For this review, take the finished solid that the model builds, in its own axes (mm). Face numbers are marked on the shaded views. Round coordinates to 2 decimals unless told otherwise and drop trailing zeros. Loops run counter-clockwise (first coordinate to the right, second up) from the corner with the lowest first, then second, coordinate; pieces in that order, holes last. Notation, with made-up numbers: (-14.75, -23) -> (28.25, -23) arc R20 ccw to (28.25, 8) -> close; hole circle Ø2 at (-13.5, -18). An arc over 180 degrees is marked (long way). Write each question's results on one line, items separated by ' | '.
```python
from build123d import *

# Parameters (mm, degrees)
BOSS_EXTRUDE1_DEPTH      = 3.75
BOSS_EXTRUDE1_DEPTH_BACK = 3.75
SKETCH1_R                = 1.5
SKETCH3_R                = 1.5
CUT_EXTRUDE1_DEPTH       = 25.5
SKETCH4_R                = 2.75
CUT_EXTRUDE2_DEPTH       = 25
CUT_EXTRUDE3_DEPTH       = 25
CUT_EXTRUDE4_DEPTH       = 3


with BuildPart() as part:
    # Sketch1 → Boss-Extrude1 (new, two sides: drawn at the far end of the back side and taken through both)
    with BuildSketch(Plane(origin=(0, 0, 0), x_dir=(0, 0, -1), z_dir=(1, 0, 0)).offset(-BOSS_EXTRUDE1_DEPTH_BACK)):
        with BuildLine():
            Line((0, 26), (0, 36))
            ThreePointArc((0, 36), (-36, 0), (0, -36))
            Line((0, -36), (0, -26))
            ThreePointArc((0, -26), (-24.020867845, -9.949769241), (-18.384776311, 18.384776311))
            ThreePointArc((-18.384776311, 18.384776311), (-9.949769241, 24.020867845), (0, 26))
        make_face()
        with Locations((-19.798989873, -19.798989873)):
            Circle(SKETCH1_R, mode=Mode.SUBTRACT)
        with BuildLine():
            ThreePointArc((-18.298989873, 19.798989873), (-18.413170574, 19.224964725), (-18.738329701, 18.738329701))
            ThreePointArc((-18.738329701, 18.738329701), (-21.184809172, 20.373015022), (-18.298989873, 19.798989873))
        make_face(mode=Mode.SUBTRACT)
    extrude(amount=BOSS_EXTRUDE1_DEPTH + BOSS_EXTRUDE1_DEPTH_BACK)

    # Sketch3 → Cut-Extrude1 (cut)
    with BuildSketch(Plane(origin=(0, 0, 0), x_dir=(-1, 0, 0), z_dir=(0, 0, -1))):
        with Locations((0, 31)):
            Circle(SKETCH3_R)
    cut_extrude1 = extrude(amount=-CUT_EXTRUDE1_DEPTH, mode=Mode.SUBTRACT)

    # Mirror1: Cut-Extrude1 across plane
    add(cut_extrude1.mirror(Plane.ZX), mode=Mode.SUBTRACT)

    # Sketch4 → Cut-Extrude2 (cut)
    with BuildSketch(Plane(origin=(0, 0, 30), x_dir=(-1, 0, 0), z_dir=(0, 0, -1))):
        with Locations(Location((0, 31, 0), (0, 0, 180))):
            Circle(SKETCH4_R)
    extrude(amount=CUT_EXTRUDE2_DEPTH, mode=Mode.SUBTRACT)

    # Sketch5 → Cut-Extrude3 (cut)
    with BuildSketch(Plane(origin=(0, 0, 30), x_dir=(-1, 0, 0), z_dir=(0, 0, -1))):
        Polygon((2.75, -32.58771324), (2.75, -29.41228676), (0, -27.824573519), (-2.75, -29.41228676), (-2.75, -32.58771324), (0, -34.175426481), align=None)
    extrude(amount=CUT_EXTRUDE3_DEPTH, mode=Mode.SUBTRACT)

    # Sketch6 → Cut-Extrude4 (cut)
    with BuildSketch(Plane(origin=(3.75, 0, 0), x_dir=(0, 0, -1), z_dir=(1, 0, 0))):
        Polygon((-22.45221952, -18.054367916), (-22.636491632, -21.224443171), (-19.983261985, -22.969065128), (-17.145760226, -21.543611831), (-16.961488115, -18.373536576), (-19.614717761, -16.628914618), align=None)
        Polygon((-18.054367916, 22.45221952), (-21.224443171, 22.636491632), (-22.969065128, 19.983261985), (-21.543611831, 17.145760226), (-18.373536576, 16.961488115), (-16.628914618, 19.614717761), align=None)
        Polygon((18.054367916, -22.45221952), (21.224443171, -22.636491632), (22.969065128, -19.983261985), (21.543611831, -17.145760226), (18.373536576, -16.961488115), (16.628914618, -19.614717761), align=None)
        Polygon((22.45221952, 18.054367916), (22.636491632, 21.224443171), (19.983261985, 22.969065128), (17.145760226, 21.543611831), (16.961488115, 18.373536576), (19.614717761, 16.628914618), align=None)
    extrude(amount=-CUT_EXTRUDE4_DEPTH, mode=Mode.SUBTRACT)


solid = part.part
```
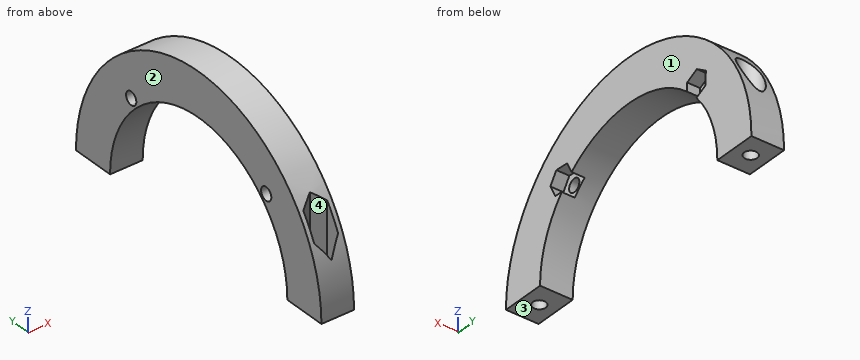
1. Consider section A-A (z = 9). State the section outline as (x, y) points, plus the area to 3 significant figures.
Values found:
outline: (-3.75, -34.86) -> (3.75, -34.86) -> (3.75, -24.39) -> (-3.75, -24.39) -> close; (-3.75, 24.39) -> (3.75, 24.39) -> (3.75, 34.86) -> (-3.75, 34.86) -> close; hole (-2.75, -32.59) -> (0, -34.18) -> (2.75, -32.59) -> (2.75, -29.41) -> (0, -27.82) -> (-2.75, -29.41) -> close; hole circle Ø5.5 at (0, 31) | area: 107 mm2
2. Consider section D-D (y = 0). State the section outline as (x, z) points, plus the area to 3 significant figures.
Values found:
outline: (-3.75, 26) -> (3.75, 26) -> (3.75, 36) -> (-3.75, 36) -> close | area: 75.0 mm2
3. To check wall thickness, follow probe 1 along X at (y, z) = (-31, 3.95); probe 2 along X at (y, z) = (31, 11); probe 3 along Y at (x, z) = (0, 2.15). State the ranges of each line that lie inside material, in increasing order.
Values found:
probe 1: x = -3.75 to -1.5, 1.5 to 3.75 | probe 2: x = -3.75 to -2.75, 2.75 to 3.75 | probe 3: y = -35.94 to -32.5, -29.5 to -25.91, 25.91 to 29.5, 32.5 to 35.94
4. For pin 1 (2.5 mm diameter, centred on y = -19.8, z = 19.8, fed in from -X); pin 2 (3 mm diameter, centred on x = -2.5, y = 7.5, fed in from +Z); pin 3 (1.6 mm diameter, centred on x = 1.5, y = -31.5, fed in from +Z); pin 4 (1.5 mm diameter, centred on x = 3, z = 29.5, fed in from -Y), all flat-tipped, find the tip position at first contact; note any pin that passes through.
Values found:
pin 1: passes through | pin 2: stops at z = 35.5 | pin 3: stops at z = 5 | pin 4: stops at y = -21.67
5. Draft analysis for pull direction X (two halves, no side actions). For the marked faces 1, 2, 3 and 4, state which applies: released by +X, released by -X, zero draft, split by the parting line, or undercut.
Values found:
face 1: released by +X | face 2: released by -X | face 3: zero draft | face 4: undercut
6. Consider section C-C (z = 14.5). State the section outline as (x, y) points.
Values found:
outline: (-3.75, -32.95) -> (-2.12, -32.95) -> (-2.75, -32.59) -> (-2.75, -29.41) -> (0, -27.82) -> (2.75, -29.41) -> (2.75, -32.59) -> (2.12, -32.95) -> (3.75, -32.95) -> (3.75, -21.58) -> (-3.75, -21.58) -> close; (-3.75, 21.58) -> (3.75, 21.58) -> (3.75, 32.95) -> (1.94, 32.95) arc R2.75 cw (long way) to (-1.94, 32.95) -> (-3.75, 32.95) -> close
7. Consider section B-B (y = 31). State the section outline as (x, z) points, plus the area to 3 significant figures.
Values found:
outline: (-3.75, 0) -> (-1.5, 0) -> (-1.5, 5) -> (-2.75, 5) -> (-2.75, 18.3) -> (-3.75, 18.3) -> close; (1.5, 0) -> (3.75, 0) -> (3.75, 18.3) -> (2.75, 18.3) -> (2.75, 5) -> (1.5, 5) -> close | area: 49.1 mm2
